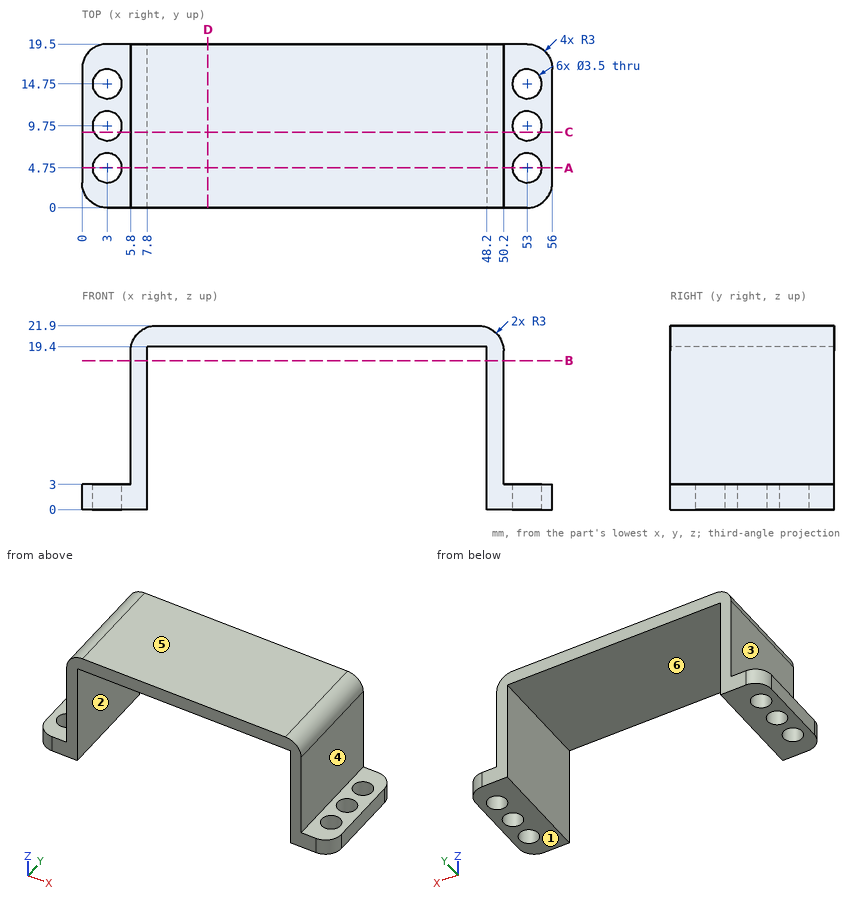
Job drawing, mm, ordinate dimensions from the low corner. One solid piece. A direction names the side the tool comes from. Round coordinates to 2 decimals unless told otherwise and drop trailing zeros. Order: outer loops, then holes, each group sorted by start corner. A loop starts at its lowest first (then second) coordinate and runs counter-clockwise, first axis right, second up. Notation, with made-up numbers: M -37,45.25 L 22,45.25 A5 ccw 22,50.25 Z; hole C 29,-15 d5. An arc over 180 degrees is marked long. Write each question's results on one line, items separated by ' | '. Start each with the question number.
(1) Which spindle directions (+Z, -Z, +X, -X, +Y, -Y) get a long thin tool onto all of the face, cutting with end or side? Do the marked faces 1, 2 and 3. Say none if no direction does.
(2) Drop flat-ended pins along their axis: pin 1 (4.5 mm diameter, centred on x = 3.5, y = 11.5, fed in from +Z); pin 2 (6 mm diameter, centred on x = 8.5, z = 7, fed in from -Y); pin 3 (8 mm diameter, centred on y = 7.5, z = 11.5, fed in from +X); pin 4 (10 mm diameter, centred on x = 21, y = 8, fed in from -Z). Give the stop position or say it passes through.
(3) Saw through at D-D, the plane x = 15. Give the cut face in (y, z), then the cut area to 4 significant figures.
(4) Saw through at A-A, the plane y = 4.75. Give the cut face in (x, z), then the cut area to 3 significant figures.
(5) Saw through at C-C, the plane y = 9. Give the cut face in (x, z), then the cut area to 3 significant figures.
(6) Two-plate mould, pull along X, no slides. Class the marked faces 4, 5 and 6: pulls with the +X half, pulls with the -X half, needs draft (parallel to the pull), parting line crosses it, or undercut.
(7) Saw through at B-B, the plane z = 17.75. Give the cut face in (x, y), then the cut area to 3 significant figures.
(8) Probe probe 1 along Y at (x, z) = (3, 1.05); probe 2 along X at (y, z) = (14.25, 14.25); probe 3 along X at (y, z) = (10.75, 2). List the from-to ranges inside material, lowest first. Write a range as from..to.
Established:
1) face 1: -Z, +X, -X, +Y, -Y | face 2: -Z, +Y, -Y | face 3: +Z, -X, +Y, -Y
2) pin 1: stops at z = 3 | pin 2: stops at y = 0 | pin 3: stops at x = 50.2 | pin 4: stops at z = 19.4
3) outline: M 0,19.4 L 19.5,19.4 L 19.5,21.9 L 0,21.9 Z | area: 48.75 mm^2
4) outline: M 0,0 L 1.25,0 L 1.25,3 L 0,3 Z; M 4.75,0 L 7.8,0 L 7.8,19.4 L 48.2,19.4 L 48.2,0 L 51.25,0 L 51.25,3 L 50.2,3 L 50.2,18.9 A3 ccw 47.2,21.9 L 8.8,21.9 A3 ccw 5.8,18.9 L 5.8,3 L 4.75,3 Z; M 54.75,0 L 56,0 L 56,3 L 54.75,3 Z | area: 199 mm^2
5) outline: M 0,0 L 1.42,0 L 1.42,3 L 0,3 Z; M 4.58,0 L 7.8,0 L 7.8,19.4 L 48.2,19.4 L 48.2,0 L 51.42,0 L 51.42,3 L 50.2,3 L 50.2,18.9 A3 ccw 47.2,21.9 L 8.8,21.9 A3 ccw 5.8,18.9 L 5.8,3 L 4.58,3 Z; M 54.58,0 L 56,0 L 56,3 L 54.58,3 Z | area: 201 mm^2
6) face 4: pulls with the +X half | face 5: needs draft | face 6: undercut
7) outline: M 5.8,0 L 7.8,0 L 7.8,19.5 L 5.8,19.5 Z; M 48.2,0 L 50.2,0 L 50.2,19.5 L 48.2,19.5 Z | area: 78.0 mm^2
8) probe 1: y = 0..3, 6.5..8, 11.5..13, 16.5..19.5 | probe 2: x = 5.8..7.8, 48.2..50.2 | probe 3: x = 0..1.56, 4.44..7.8, 48.2..51.56, 54.44..56
